```python
from build123d import *

# Parameters (mm, degrees)
SKETCH1_R           = 1.5875
BOSS_EXTRUDE1_DEPTH = 2.54
BOSS_EXTRUDE2_DEPTH = 8.255
SKETCH3_W           = 64.77
SKETCH3_H           = 7.1
CUT_EXTRUDE1_DEPTH  = 0.635
SKETCH9_R           = 1.5875
CUT_EXTRUDE4_DEPTH  = 3.54
SKETCH4_R           = 1.143
CUT_EXTRUDE2_DEPTH  = 11.43
BOSS_EXTRUDE5_DEPTH = 8.255
SKETCH28_R          = 1.5875
CUT_EXTRUDE12_DEPTH = 7.62
SKETCH29_R          = 1.5875
CUT_EXTRUDE13_DEPTH = 10.16
SKETCH30_R          = 1.5875
CUT_EXTRUDE14_DEPTH = 12.7
SKETCH31_R          = 1.5875
CUT_EXTRUDE15_DEPTH = 12.7
SKETCH32_R          = 1.5875
CUT_EXTRUDE16_DEPTH = 12.7
BOSS_EXTRUDE6_DEPTH = 2.54
CUT_EXTRUDE17_DEPTH = 3.5400001


with BuildPart() as part:
    # Sketch1 → Boss-Extrude1 (new body)
    with BuildSketch(Plane.XY):
        with BuildLine():
            Line((-71.572584947, 25.4), (-65.222584947, 25.4))
            Line((-65.222584947, 25.4), (-65.222584947, 22.86))
            ThreePointArc((-65.222584947, 22.86), (-63.362713008, 18.369871939), (-58.872584947, 16.51))
            Line((-58.872584947, 16.51), (44.196, 16.51))
            ThreePointArc((44.196, 16.51), (48.686128061, 18.369871939), (50.546, 22.86))
            Line((50.546, 22.86), (50.546, 44.45))
            Line((50.546, 44.45), (61.579155694, 44.45))
            ThreePointArc((61.579155694, 44.45), (75.946, 0), (61.579155694, -44.45))
            Line((61.579155694, -44.45), (50.546, -44.45))
            Line((50.546, -44.45), (50.546, -22.86))
            ThreePointArc((50.546, -22.86), (48.686128061, -18.369871939), (44.196, -16.51))
            Line((44.196, -16.51), (-58.872584947, -16.51))
            ThreePointArc((-58.872584947, -16.51), (-63.362713008, -18.369871939), (-65.222584947, -22.86))
            Line((-65.222584947, -22.86), (-65.222584947, -25.4))
            Line((-65.222584947, -25.4), (-71.572584947, -25.4))
            ThreePointArc((-71.572584947, -25.4), (-75.946, 0), (-71.572584947, 25.4))
        make_face()
        with Locations((-45.72, 8.128)):
            Circle(SKETCH1_R, mode=Mode.SUBTRACT)
        with Locations((-45.72, -8.128)):
            Circle(SKETCH1_R, mode=Mode.SUBTRACT)
    extrude(amount=BOSS_EXTRUDE1_DEPTH)

    # Sketch2 → Boss-Extrude2 (add)
    with BuildSketch(Plane.XY.offset(2.54)):
        with BuildLine():
            Line((61.865268471, 17.78), (60.095110466, 38.1))
            ThreePointArc((60.095110466, 38.1), (59.464196764, 40.158289632), (58.047089349, 41.778911391))
            Line((58.047089349, 41.778911391), (57.900800643, 44.704))
            Line((57.900800643, 44.704), (61.395010384, 44.704))
            ThreePointArc((61.395010384, 44.704), (69.822038137, 29.877715884), (74.728381149, 13.544887112))
            Line((74.728381149, 13.544887112), (60.759450402, 13.544887112))
            Line((60.759450402, 13.544887112), (60.759450402, 15.094127876))
            ThreePointArc((60.759450402, 15.094127876), (61.639191639, 16.302501703), (61.865268471, 17.78))
        make_face()
        with BuildLine():
            Line((58.651639318, 17.500047669), (56.881481313, 37.820047669))
            Line((56.881481313, 37.820047669), (50.546, 37.820047669))
            Line((50.546, 37.820047669), (50.546, 16.566735288))
            Line((50.546, 16.566735288), (57.366094516, 16.566735288))
            ThreePointArc((57.366094516, 16.566735288), (58.160401987, 16.824667019), (58.651639318, 17.500047669))
        make_face()
        with BuildLine():
            Line((60.759450402, -13.544887112), (74.728381149, -13.544887112))
            ThreePointArc((74.728381149, -13.544887112), (69.822038137, -29.877715884), (61.395010384, -44.704))
            Line((61.395010384, -44.704), (57.900800643, -44.704))
            Line((57.900800643, -44.704), (58.047089349, -41.778911391))
            ThreePointArc((58.047089349, -41.778911391), (59.464196764, -40.158289632), (60.095110466, -38.1))
            Line((60.095110466, -38.1), (61.865268471, -17.78))
            ThreePointArc((61.865268471, -17.78), (61.639191639, -16.302501703), (60.759450402, -15.094127876))
            Line((60.759450402, -15.094127876), (60.759450402, -13.544887112))
        make_face()
        with BuildLine():
            Line((50.546, -16.566735288), (57.366094516, -16.566735288))
            ThreePointArc((57.366094516, -16.566735288), (58.160401987, -16.824667019), (58.651639318, -17.500047669))
            Line((58.651639318, -17.500047669), (56.881481313, -37.820047669))
            Line((56.881481313, -37.820047669), (50.546, -37.820047669))
            Line((50.546, -37.820047669), (50.546, -16.566735288))
        make_face()
    extrude(amount=BOSS_EXTRUDE2_DEPTH)

    # Sketch3 → Cut-Extrude1 (cut)
    with BuildSketch(Plane.XY.offset(2.54)):
        with Locations((44.577, 0)):
            Rectangle(SKETCH3_W, SKETCH3_H)
    extrude(amount=-CUT_EXTRUDE1_DEPTH, mode=Mode.SUBTRACT)

    # Sketch9 → Cut-Extrude4 (cut, through all)
    with BuildSketch(Plane.XY.offset(2.54)):
        with Locations((7.62, -7.239)):
            Circle(SKETCH9_R)
        with Locations((7.62, 7.239)):
            Circle(SKETCH9_R)
    extrude(amount=-CUT_EXTRUDE4_DEPTH, mode=Mode.SUBTRACT)

    # Sketch4 → Cut-Extrude2 (cut)
    with BuildSketch(Plane.XY.offset(1.905)):
        with Locations((19.812, 0)):
            Circle(SKETCH4_R)
        with Locations((34.798, 0)):
            Circle(SKETCH4_R)
        with Locations((49.784, 0)):
            Circle(SKETCH4_R)
        with Locations((64.77, 0)):
            Circle(SKETCH4_R)
    extrude(amount=-CUT_EXTRUDE2_DEPTH, mode=Mode.SUBTRACT)

    # Sketch19 → Boss-Extrude5 (add)
    with BuildSketch(Plane.XY.offset(2.54)):
        with BuildLine():
            Line((-71.572584947, -25.4), (-65.222584947, -25.4))
            Line((-65.222584947, -25.4), (-65.222584947, 25.4))
            Line((-65.222584947, 25.4), (-71.572584947, 25.4))
            ThreePointArc((-71.572584947, 25.4), (-75.946, 0), (-71.572584947, -25.4))
        make_face()
    extrude(amount=BOSS_EXTRUDE5_DEPTH)

    # Sketch28 → Cut-Extrude12 (cut)
    with BuildSketch(Plane(origin=(65.771165316, 37.973, 0), x_dir=(0, 0, -1), z_dir=(0.866025404, 0.5, 0))):
        with Locations((-6.053310192, 0)):
            Circle(SKETCH28_R)
    cut_extrude12 = extrude(amount=-CUT_EXTRUDE12_DEPTH, mode=Mode.SUBTRACT)

    # Sketch29 → Cut-Extrude13 (cut)
    with BuildSketch(Plane(origin=(73.358202803, 19.656271199, 0), x_dir=(0, 0, -1), z_dir=(0.965925826, 0.258819045, 0))):
        with Locations((-6.096, 0)):
            Circle(SKETCH29_R)
    cut_extrude13 = extrude(amount=-CUT_EXTRUDE13_DEPTH, mode=Mode.SUBTRACT)

    # Mirror3: Cut-Extrude12, Cut-Extrude13 across plane
    add(cut_extrude12.mirror(Plane.ZX), mode=Mode.SUBTRACT)
    add(cut_extrude13.mirror(Plane.ZX), mode=Mode.SUBTRACT)

    # Sketch30 → Cut-Extrude14 (cut)
    with BuildSketch(Plane(origin=(-73.358202803, 19.656271199, 0), x_dir=(0, 0, 1), z_dir=(-0.965925826, 0.258819045, 0))):
        with Locations((6.096, 0)):
            Circle(SKETCH30_R)
    extrude(amount=-CUT_EXTRUDE14_DEPTH, mode=Mode.SUBTRACT)

    # Sketch31 → Cut-Extrude15 (cut)
    with BuildSketch(Plane.ZY.offset(75.946)):
        with Locations((6.096, 0)):
            Circle(SKETCH31_R)
    extrude(amount=-CUT_EXTRUDE15_DEPTH, mode=Mode.SUBTRACT)

    # Sketch32 → Cut-Extrude16 (cut)
    with BuildSketch(Plane(origin=(-73.358202803, -19.656271199, 0), x_dir=(0, 0, 1), z_dir=(-0.965925826, -0.258819045, 0))):
        with Locations((6.096, 0)):
            Circle(SKETCH32_R)
    extrude(amount=-CUT_EXTRUDE16_DEPTH, mode=Mode.SUBTRACT)

    # Sketch33 → Boss-Extrude6 (add)
    with BuildSketch(Plane.XY.offset(2.54)):
        with BuildLine():
            Line((12.137284041, 16.51), (-58.872584947, 16.51))
            ThreePointArc((-58.872584947, 16.51), (-63.362713008, 18.369871939), (-65.222584947, 22.86))
            Line((-65.222584947, 22.86), (-65.222584947, 7.62))
            ThreePointArc((-65.222584947, 7.62), (-63.362713008, 12.110128061), (-58.872584947, 13.97))
            Line((-58.872584947, 13.97), (12.137284041, 13.97))
            Line((12.137284041, 13.97), (12.137284041, 16.51))
        make_face()
        with BuildLine():
            Line((12.137284041, -13.97), (12.137284041, -16.51))
            Line((12.137284041, -16.51), (-58.872584947, -16.51))
            ThreePointArc((-58.872584947, -16.51), (-63.362713008, -18.369871939), (-65.222584947, -22.86))
            Line((-65.222584947, -22.86), (-65.222584947, -7.62))
            ThreePointArc((-65.222584947, -7.62), (-63.362713008, -12.110128061), (-58.872584947, -13.97))
            Line((-58.872584947, -13.97), (12.137284041, -13.97))
        make_face()
    extrude(amount=BOSS_EXTRUDE6_DEPTH)

    # Sketch34 → Cut-Extrude17 (cut, through all)
    with BuildSketch(Plane.XY.offset(2.54)):
        with BuildLine():
            Line((-33.472584947, 10.16), (-5.532584947, 10.16))
            ThreePointArc((-5.532584947, 10.16), (-1.042456886, 8.300128061), (0.817415053, 3.81))
            Line((0.817415053, 3.81), (0.817415053, -3.81))
            ThreePointArc((0.817415053, -3.81), (-1.042456886, -8.300128061), (-5.532584947, -10.16))
            Line((-5.532584947, -10.16), (-34.039131073, -10.16))
            ThreePointArc((-34.039131073, -10.16), (-38.158738375, -8.120468891), (-39.822584947, -3.83532408))
            Line((-39.822584947, -3.83532408), (-39.822584947, 3.81))
            ThreePointArc((-39.822584947, 3.81), (-37.962713008, 8.300128061), (-33.472584947, 10.16))
        make_face()
    extrude(amount=-CUT_EXTRUDE17_DEPTH, mode=Mode.SUBTRACT)


solid = part.part
```
Verification items for the finished model (mm, model axes). A direction names the side the tool comes from. Coordinates: 2 decimals unless noted, no trailing zeros. Loops run counter-clockwise (first coordinate to the right, second up) from the corner with the lowest first, then second, coordinate; pieces in that order, holes last. Notation, with made-up numbers: (-28, -10) -> (18, -10) arc R28 ccw to (18, 27) -> close; hole circle Ø5 at (30, 52.5). An arc over 180 degrees is marked (long way). Put each result on its own line as item: value.
1. Gauge pin test, flat ends, axial feed: P1, Ø0.8, axis at x = -19, z = 1.5, coming from the -Y side; P2, Ø0.5, axis at y = -14.5, z = 8.5, coming from the -X side; P3, Ø3, axis at y = -0.5, z = 1.5, coming from the -X side. Record the tip position at first contact, or that the pin passes through.
Result set:
P1: stops at y = -16.51
P2: stops at x = -74.6
P3: stops at x = -75.95
2. Section check B-B, the plane x = -45.72. Record the boundary of the cut face in (y, z).
Result set:
outline: (-16.51, 0) -> (-9.72, 0) -> (-9.72, 2.54) -> (-13.97, 2.54) -> (-13.97, 5.08) -> (-16.51, 5.08) -> close; (-6.54, 0) -> (6.54, 0) -> (6.54, 2.54) -> (-6.54, 2.54) -> close; (9.72, 0) -> (16.51, 0) -> (16.51, 5.08) -> (13.97, 5.08) -> (13.97, 2.54) -> (9.72, 2.54) -> close
3. Tool access check on faces 4 (the face through (57.973, -43.262, 6.61)), 5 (the face through (-63.31, -18.32, 2.5)), 6 (the face through (60.993, 27.798, 6.61)). Record the directions out of +Z, -Z, +X, -X, +Y, -Y that give a thin tool (end or side, any length) a straight path to the whole face; none if there is none.
Result set:
face 4: +Z, -X
face 5: +Z, -Z, -Y
face 6: +Z
4. Section check A-A, the plane x = -8. Record the boundary of the cut face in (y, z), then the cut area to 3 significant figures.
Result set:
outline: (-16.51, 0) -> (-10.16, 0) -> (-10.16, 2.54) -> (-13.97, 2.54) -> (-13.97, 5.08) -> (-16.51, 5.08) -> close; (10.16, 0) -> (16.51, 0) -> (16.51, 5.08) -> (13.97, 5.08) -> (13.97, 2.54) -> (10.16, 2.54) -> close
area: 45.2 mm^2
5. Thickness scan on line 1 (Y direction, x = 7.62, z = 1.35); line 2 (Y direction, x = -45.72, z = 0.8); line 3 (Z direction, x = -68, y = 0) (1 decimal). Record the ranges inside material, lowest first.
Result set:
line 1: y = -16.51 to -8.83, -5.65 to 5.65, 8.83 to 16.51
line 2: y = -16.51 to -9.72, -6.54 to 6.54, 9.72 to 16.51
line 3: z = 0 to 4.5, 7.7 to 10.8
6. Mould release check, pull along Y, two halves, no side actions. Record for faces 1 (the face through (60.97, -28.08, 6.61)), 2 (the face through (50.546, -28, 5)), 3 (the face through (60, 44.704, 7)): pulls with the +Y half, pulls with the -Y half, needs draft (parallel to the pull), parting line crosses it, or undercut.
Result set:
face 1: undercut
face 2: needs draft
face 3: pulls with the +Y half
